```python
from build123d import *

# Parameters (mm, degrees)
F0_W     = 275
F0_H     = 70
F1_DEPTH = 35
F2_W     = 70
F2_H     = 17.5
F3_DEPTH = 70.001
F5_DEPTH = 35.001
F7_DEPTH = 17.5


with BuildPart() as f1:
    # F0 (on Front) → F1 (new body)
    with BuildSketch(Plane.XZ):
        with Locations((137.5, 35)):
            Rectangle(F0_W, F0_H)
    extrude(amount=F1_DEPTH)

    # F2 (on face) → F3 (cut, through all)
    with BuildSketch(Plane(origin=(0, 0, 0), x_dir=(1, 0, 0), z_dir=(0, 0, -1))):
        with Locations((240, 26.25)):
            Rectangle(F2_W, F2_H)
    extrude(amount=-F3_DEPTH, mode=Mode.SUBTRACT)

    # F4 (on face) → F5 (cut, through all)
    with BuildSketch(Plane.XZ.offset(35)):
        Polygon((40.58855, 0), (0, 35), (0, 0), align=None)
    extrude(amount=-F5_DEPTH, mode=Mode.SUBTRACT)

    # F6 (on face) → F7 (cut)
    with BuildSketch(Plane.XZ.offset(35)):
        Polygon((40.58855, 0), (122.794275, 0), (41.617175, 70), (0, 70), (0, 35), align=None)
    extrude(amount=-F7_DEPTH, mode=Mode.SUBTRACT)


solid = f1.part
```
Input: part model. Units: mm. Frame: model coordinates. A direction names the side the tool comes from. Coordinates: 2 decimals unless noted, no trailing zeros. Write each loop counter-clockwise with the first axis right and the second up, starting at its lowest first coordinate (ties: lowest second). Pieces come first, ordered by that corner, then holes. Notation, with made-up numbers: (81, 45) -> (109, 45) arc R22 cw to (109, 73) -> close; hole circle Ø2 at (29.5, -16.5). An arc over 180 degrees is marked (long way). Answer as a JSON object with one key per item and string values.
1. Section D-D on z = 19.5. Return the cut outline in (x, y).
Result set:
{"outline": "(17.97, -17.5) -> (100.18, -17.5) -> (100.18, -35) -> (205, -35) -> (205, -17.5) -> (275, -17.5) -> (275, 0) -> (17.97, 0) -> close"}
2. First-contact query: P1, Ø5, axis at y = -27, z = 44, coming from the +X side; P2, Ø10, axis at x = 141, y = -25, coming from the -Z side; P3, Ø1, axis at x = 58.5, z = 54, coming from the -Y side. Flat tips, straight axial feed; report the tip coordinate or a pass-through.
Result set:
{"P1": "stops at x = 205", "P2": "stops at z = 0", "P3": "stops at y = -17.5"}
3. Access query for faces 1 (the face through (82.774, -26.373, 34.51)), 2 (the face through (136, -17, 70)), 3 (the face through (205, -26, 35)). Directions: +Z, -Z, +X, -X, +Y, -Y. A direction counts if a zero-diameter tool reaches every point of the face in a straight line with its end or side. Return the directions, or none.
Result set:
{"face 1": "-Z, -X, -Y", "face 2": "+Z, +X, -X, +Y, -Y", "face 3": "+Z, -Z, +X, -Y"}
4. Section C-C on y = -13. Return the cut outline in (x, z), then the cut area to 3 significant figures.
Result set:
{"outline": "(0, 35) -> (40.59, 0) -> (275, 0) -> (275, 70) -> (0, 70) -> close", "area": "18,500 mm2"}
5. Section A-A on z = 50. Return the cut outline in (x, y).
Result set:
{"outline": "(0, -17.5) -> (64.81, -17.5) -> (64.81, -35) -> (205, -35) -> (205, -17.5) -> (275, -17.5) -> (275, 0) -> (0, 0) -> close"}
6. Material intervals for line 1 (Y direction, x = 260, z = 48); line 2 (X direction, y = -22, z = 34); line 3 (X direction, y = -30, z = 9), sorted ascending. Write a range as from..to.
Result set:
{"line 1": "y = -17.5..0", "line 2": "x = 83.37..205", "line 3": "x = 112.36..205"}
7. Section B-B on x = 254. Return the cut outline in (y, z), then the cut area to 4 significant figures.
Result set:
{"outline": "(-17.5, 0) -> (0, 0) -> (0, 70) -> (-17.5, 70) -> close", "area": "1,225 mm2"}
